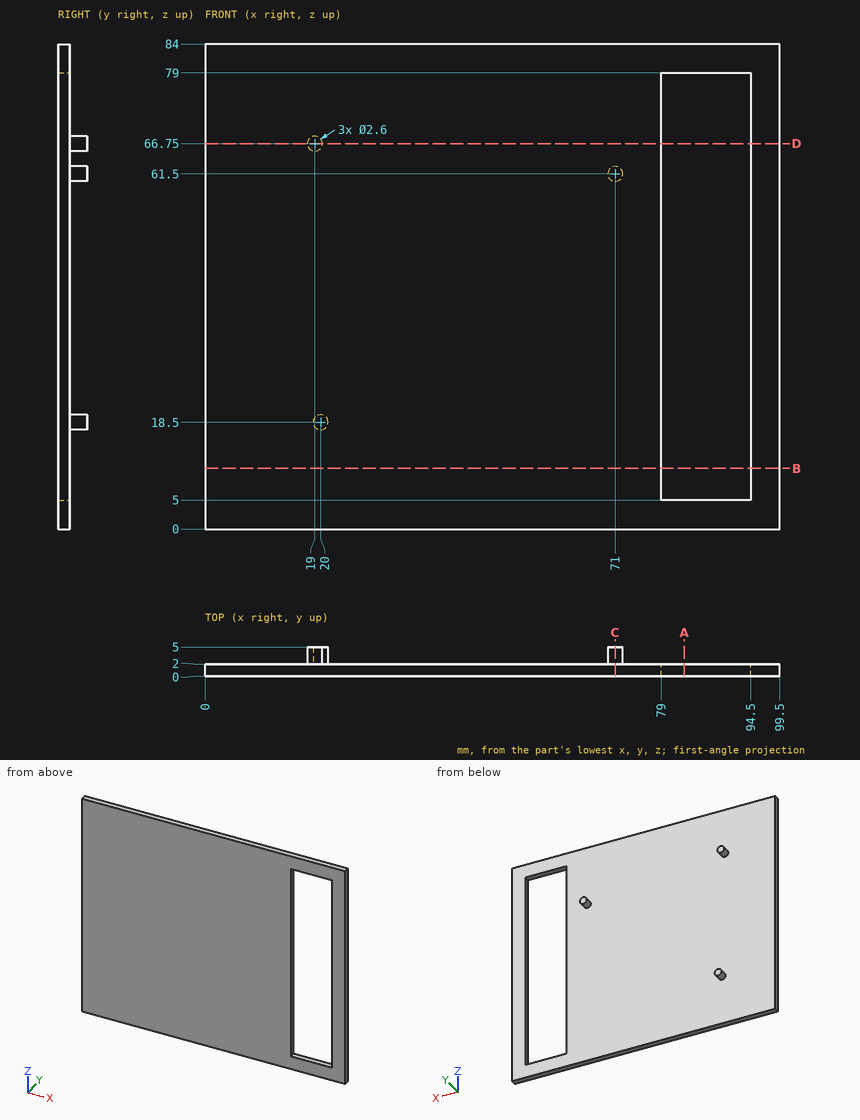
The figure shows three views and two pictorial views of one solid part (mm, origin at its lowest corner). Answer the questions. Coordinates: 2 decimals unless noted, no trailing zeros. Loops run counter-clockwise (first coordinate to the right, second up) from the corner with the lowest first, then second, coordinate; pieces in that order, holes last. Notation, with made-up numbers: M -20,34 L 27,34 A14 ccw 27,58 Z; hole C 30,-3 d6. An arc over 180 degrees is marked long. Use CSV: the item, a comma, the result in double quotes. Start each with the question number.
(1) Find section D-D, the plane z = 66.75. Give the vertices of the cut face in (x, y).
(2) Find section A-A, the plane x = 83. Give the vertices of the cut face in (y, z).
(3) Given pin 1 Ø1 at (x, z) = (15.5, 14.5) entering from +Y, flat-ended and moving along its own axis, determine where the tip first touches the part or whether it passes through.
(4) Find section B-B, the plane z = 10.5. Give the vertices of the cut face in (x, y).
(5) Find section C-C, the plane x = 71. Give the vertices of the cut face in (y, z), then the cut area to 3 significant figures.
(6) Consider line 1 (X direction, y = 0.25, z = 13); line 2 (Y direction, x = 77, z = 36). Determine where each line is inside the solid, lowest interval first.
Recorded:
1,outline,"M 0,0 L 79,0 L 79,2 L 20.3,2 L 20.3,5 L 17.7,5 L 17.7,2 L 0,2 Z; M 94.5,0 L 99.5,0 L 99.5,2 L 94.5,2 Z"
2,outline,"M 0,0 L 2,0 L 2,5 L 0,5 Z; M 0,79 L 2,79 L 2,84 L 0,84 Z"
3,pin 1,"stops at y = 2"
4,outline,"M 0,0 L 79,0 L 79,2 L 0,2 Z; M 94.5,0 L 99.5,0 L 99.5,2 L 94.5,2 Z"
5,outline,"M 0,0 L 2,0 L 2,60.2 L 5,60.2 L 5,62.8 L 2,62.8 L 2,84 L 0,84 Z"
5,area,"176 mm^2"
6,line 1,"x = 0 to 79, 94.5 to 99.5"
6,line 2,"y = 0 to 2"
